Autodesk Inventor part; units mm, degrees
ref_plane "YZ Plane" through (0, 0, 0) normal (1, 0, 0) x (0, 1, 0)
ref_plane "XZ Plane" through (0, 0, 0) normal (0, 1, 0) x (-1, 0, 0)
ref_plane "XY Plane" through (0, 0, 0) normal (0, 0, 1) x (1, 0, 0)
sketch "Sketch1" plane through (0, 0, 0) normal (0, 0, 1) x (1, 0, 0)
  line L0 (2.7496, 4.7625) -> (5.4993, 0)
  line L1 (5.4993, 0) -> (2.7496, -4.7625)
  line L2 (2.7496, -4.7625) -> (-2.7496, -4.7625)
  line L3 (-2.7496, -4.7625) -> (-5.4993, 0)
  line L4 (-5.4993, 0) -> (-2.7496, 4.7625)
  line L5 (-2.7496, 4.7625) -> (2.7496, 4.7625)
  circle A0 centre (0, 0) radius 7.9375
  circle A1 centre (0, 0) radius 5.4993 construction
  dimension "d0" = 9.525
  dimension "d2" = 15.875
  dimension "d3" = 2.4382
extrude "Extrusion1" add sketch "Sketch1" against normal blind 19.05
thicken "Thicken Hex" operation add thickness 0.127 both sides no extend neighbours yes toward (-0.8660254, 0.5, 0) faces at (-4.5827, 1.5875, -6.35) (-3.6662, -3.175, -6.35) (0.9165, -4.7625, -6.35) (-0.9165, 4.7625, -6.35) (3.6662, 3.175, -6.35) (4.5827, -1.5875, -6.35)
sketch "Sketch3" plane through (0, 0, 0) normal (0, 0, 1) x (1, 0, 0)
  line L0 (5.6459, 0) -> (2.823, -4.8895)
  line L1 (2.823, -4.8895) -> (-2.823, -4.8895)
  line L2 (-2.823, -4.8895) -> (-5.6459, 0)
  line L3 (-5.6459, 0) -> (-2.823, 4.8895)
  line L4 (-2.823, 4.8895) -> (2.823, 4.8895)
  line L5 (2.823, 4.8895) -> (5.6459, 0)
  line L6 (2.823, 4.8895) -> (5.6459, 0)
  circle A0 centre (0, 0) radius 6.35
  dimension "d10" = 12.7
extrude "Extrusion2" add sketch "Sketch3" along normal blind 12.7
thicken "Thicken2" operation add thickness 0.127 both sides no extend neighbours yes toward (-0.9967573, 0.0804666, 0) faces at (6.3294, -0.511, 8.4667)
equation "\"d0\" = hexSize"
equation "\"d2\" = exteriorDiameter"
equation "\"d4\" = length"
equation "\"d6\" = printSpacing"
equation "\"d7\" = printSpacing"
equation "\"d10\" = baseBushingDiameter"
equation "\"d8\" = baseBushingLength"
equation "\"d11\" = printSpacing"
equation "\"d12\" = printSpacing"
equation "\"hexSize\" = 9.525"
equation "\"exteriorDiameter\" = 15.875"
equation "\"length\" = 19.05"
equation "\"printSpacing\" = 0.127"
equation "\"baseBushingDiameter\" = 12.7"
equation "\"baseBushingLength\" = 12.7"
properties part number "3_8x5_8x3_4-hexBearingEndCap" material "PC/ABS Plastic"
The listing builds one solid part. Answer for the finished solid, in the listing's coordinates (mm). A direction names the side the tool comes from. Round coordinates to 2 decimals unless told otherwise and drop trailing zeros. Loops run counter-clockwise (first coordinate to the right, second up) from the corner with the lowest first, then second, coordinate; pieces in that order, holes last.
1) Consider line 1 (Y direction, x = 0, z = 5.5); line 2 (Z direction, x = -7, y = -2.25); line 3 (Y direction, x = 2.25, z = 2.5). Determine where each line is inside the solid, lowest interval first.
Outcome:
line 1: y = -6.22 to -4.89, 4.89 to 6.22
line 2: z = -19.05 to 0
line 3: y = -5.8 to -4.89, 4.89 to 5.8
2) A cutting plane is placed at A-A on x = 0. Determine the outline of the cut face in (y, z).
Outcome:
outline: (-7.94, -19.05) - (-4.89, -19.05) - (-4.89, 12.7) - (-6.22, 12.7) - (-6.22, 0) - (-7.94, 0) - close; (4.89, -19.05) - (7.94, -19.05) - (7.94, 0) - (6.22, 0) - (6.22, 12.7) - (4.89, 12.7) - close
3) Given P1, Ø1, axis at x = 3, y = 1.5, coming from the +Z side; P2, Ø8, axis at x = 2.5, z = 6, coming from the +Y side; P3, Ø4, axis at y = -4.5, z = -1.5, coming from the -X side; P4, Ø4, axis at x = 3.5, z = 6, coming from the -Y side, each flat-ended and moving along its own axis, determine where each tip first touches the part or whether it passes through.
Outcome:
P1: passes through
P2: stops at y = 6.22
P3: stops at x = -7.53
P4: stops at y = -6.04
4) A cutting plane is placed at D-D on x = -4.75. Determine the outline of the cut face in (y, z), plus the area to 3 significant figures.
Outcome:
outline: (-6.36, -19.05) - (-1.55, -19.05) - (-1.55, 12.7) - (-4.02, 12.7) - (-4.02, 0) - (-6.36, 0) - close; (1.55, -19.05) - (6.36, -19.05) - (6.36, 0) - (4.02, 0) - (4.02, 12.7) - (1.55, 12.7) - close
area: 246 mm2
5) For faces 1 (the face through (-0.5, 5.1, 12.7)), 2 (the face through (0, -4.89, -3)), 3 (the face through (-1.349, 6.075, 6.261)), determine the directions among +Z, -Z, +X, -X, +Y, -Y from which every point of the face is accessible in a straight line to the end or side of a thin tool.
Outcome:
face 1: +Z, +X, -X, +Y, -Y
face 2: +Z, -Z
face 3: +Z
6) For a pull along X with two mould halves and no side action, classify faces 4 (the face through (-0.1, -5.2, -19.05)), 5 (the face through (0, 4.89, -3)), 6 (the face through (-1.72, -7.75, -9.39)) as released by +X, released by -X, zero draft, split by the parting line, or undercut.
Outcome:
face 4: zero draft
face 5: undercut
face 6: split by the parting line
7) A cutting plane is placed at B-B on y = 1.25. Determine the outline of the cut face in (x, z).
Outcome:
outline: (-7.84, -19.05) - (-4.92, -19.05) - (-4.92, 12.7) - (-6.1, 12.7) - (-6.1, 0) - (-7.84, 0) - close; (4.92, -19.05) - (7.84, -19.05) - (7.84, 0) - (6.1, 0) - (6.1, 12.7) - (4.92, 12.7) - close
8) A cutting plane is placed at C-C on z = 10.5. Determine the outline of the cut face in (x, y).
Outcome:
outline: circle Ø12.45 at (0, 0); hole (-5.65, 0) - (-2.82, -4.89) - (2.82, -4.89) - (5.65, 0) - (2.82, 4.89) - (-2.82, 4.89) - close
